from build123d import *

# Parameters (mm, degrees)
EXTRUDE_1_DEPTH     = 30
EXTRUDE_2_DEPTH     = 4
SKETCH_3_R          = 3.25
CUT_EXTRUDE_1_DEPTH = 7
SKETCH_4_W          = 2.5
SKETCH_4_H          = 6
EXTRUDE_3_DEPTH     = 2.5


with BuildPart() as part:
    # Эскиз1 → Бобышка-Вытянуть1 (new body, symmetric)
    with BuildSketch(Plane.XY):
        Polygon((0, 60), (0, 0), (60, 0), (60, 6), (6, 6), (6, 60), align=None)
    extrude(amount=EXTRUDE_1_DEPTH, both=True)

    # Эскиз2 → Бобышка-Вытянуть2 (add)
    with BuildSketch(Plane.XY.offset(30)):
        with BuildLine():
            Line((60, 6), (6, 6))
            Line((6, 6), (6, 60))
            Line((6, 60), (9, 60))
            ThreePointArc((9, 60), (11.121320344, 59.121320344), (12, 57))
            Line((12, 57), (12, 55))
            Line((12, 55), (55, 12))
            Line((55, 12), (57, 12))
            ThreePointArc((57, 12), (59.121320344, 11.121320344), (60, 9))
            Line((60, 9), (60, 6))
        make_face()
    extrude_2 = extrude(amount=-EXTRUDE_2_DEPTH)

    # Зеркальное отражение2: Бобышка-Вытянуть2 across plane
    add(extrude_2.mirror(Plane.XY))

    # Эскиз3 → Вырез-Вытянуть1 (cut, through all)
    with BuildSketch(Plane(origin=(0, 6, 0), x_dir=(1, 0, 0), z_dir=(0, 1, 0))):
        with Locations(Location((45, -15, 0), (0, 0, 270))):  # turned: the seam where the file's is
            Circle(SKETCH_3_R)
        with Locations(Location((45, 15, 0), (0, 0, 90))):  # turned: the seam where the file's is
            Circle(SKETCH_3_R)
        with BuildLine():
            Line((17, -11.75), (31, -11.75))
            ThreePointArc((31, -11.75), (34.25, -15), (31, -18.25))
            Line((31, -18.25), (17, -18.25))
            ThreePointArc((17, -18.25), (13.75, -15), (17, -11.75))
        make_face()
        with BuildLine():
            Line((17, 11.75), (31, 11.75))
            ThreePointArc((31, 11.75), (34.25, 15), (31, 18.25))
            Line((31, 18.25), (17, 18.25))
            ThreePointArc((17, 18.25), (13.75, 15), (17, 11.75))
        make_face()
    cut_extrude_1 = extrude(amount=-CUT_EXTRUDE_1_DEPTH, mode=Mode.SUBTRACT)

    # Эскиз4 → Бобышка-Вытянуть3 (add)
    with BuildSketch(Plane.XZ):
        with Locations((4.25, -15)):
            Rectangle(SKETCH_4_W, SKETCH_4_H)
        with Locations((55.75, -15)):
            Rectangle(SKETCH_4_W, SKETCH_4_H)
        with Locations((55.75, 15)):
            Rectangle(SKETCH_4_W, SKETCH_4_H)
        with Locations((4.25, 15)):
            Rectangle(SKETCH_4_W, SKETCH_4_H)
    extrude_3 = extrude(amount=EXTRUDE_3_DEPTH)

    # Зеркальное отражение3: Вырез-Вытянуть1, Бобышка-Вытянуть3 across plane
    add(cut_extrude_1.mirror(Plane(origin=(0, 0, 0), x_dir=(0, 0, 1), z_dir=(-0.707106781, 0.707106781, 0))), mode=Mode.SUBTRACT)
    add(extrude_3.mirror(Plane(origin=(0, 0, 0), x_dir=(0, 0, 1), z_dir=(-0.707106781, 0.707106781, 0))))


solid = part.part
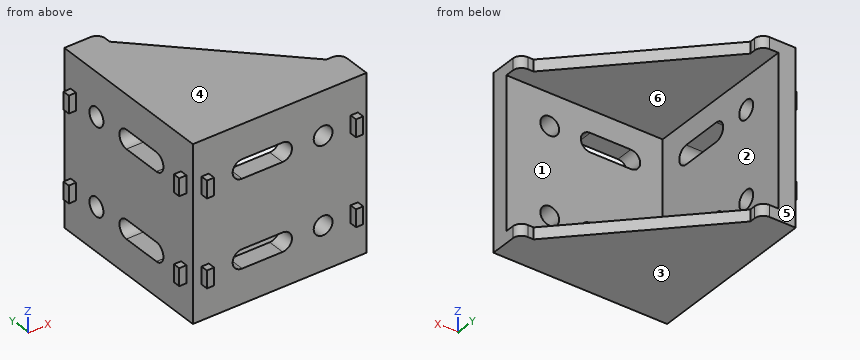
Input: part model. Units: mm. Frame: model coordinates. Face numbers are marked on the shaded views. A direction names the side the tool comes from. Coordinates: 2 decimals unless noted, no trailing zeros. Loops run counter-clockwise (first coordinate to the right, second up) from the corner with the lowest first, then second, coordinate; pieces in that order, holes last. Notation, with made-up numbers: (72.5, 2) - (89.5, 2) arc R18 ccw to (89.5, 26) - close; hole circle Ø4 at (-28.75, 88.25). An arc over 180 degrees is marked (long way). Answer in a Markdown table with one row per item. Add a question column.
Item 1: Section query A-A on x = 45. Return the cut outline in (y, z).
Item 2: Mould query, pull axis Z, two halves, no side actions, for the marked faces 1, 2, 3 and 4. Classes: released by +Z, released by -Z, zero draft, split by the parting line, or undercut.
Item 3: Section query B-B on y = 30. Return the cut outline in (x, z), then the cut area to 3 significant figures.
Item 4: Line query: line 1 along X through (y, z) = (4, 15); line 2 along Y through (x, z) = (2, -15). Output: solid intervals per line, ascending. Write a range as [from, to].
Item 5: Section query D-D on z = 15. State how many separate pieces and enclosed holes the cut face has, then the cut area to 3 significant figures.
Item 6: Section query C-C on y = 2. Return the cut outline in (x, z).
Item 7: Access query for the marked faces 5 and 6. Directions: +Z, -Z, +X, -X, +Y, -Y. A direction counts if a zero-diameter tool reaches every point of the face in a straight line with its end or side. Return the directions, or none.
Item 8: Contact query for flat-ended pins moving along their axis: P1, Ø0.8, axis at x = -1, y = 4, coming from the -Z side; P2, Ø0.8, axis at y = -1.5, z = -14.5, coming from the -X side; P3, Ø6, axis at x = 32.5, z = -10.5, coming from the +Y side. Output: stop coordinate, or through.
Recorded:
| question | item | result |
|---|---|---|
| 1 | outline | (0, -30) - (22, -30) - (22, -26) - (6, -26) - (6, -18.25) - (0, -18.25) - close; (0, -11.75) - (6, -11.75) - (6, 11.75) - (0, 11.75) - close; (0, 18.25) - (6, 18.25) - (6, 26) - (22, 26) - (22, 30) - (0, 30) - close |
| 2 | face 1 | undercut |
| 2 | face 2 | undercut |
| 2 | face 3 | released by -Z |
| 2 | face 4 | released by +Z |
| 3 | outline | (0, -30) - (37, -30) - (37, -26) - (6, -26) - (6, -18.25) - (0, -18.25) - close; (0, -11.75) - (6, -11.75) - (6, 11.75) - (0, 11.75) - close; (0, 18.25) - (6, 18.25) - (6, 26) - (37, 26) - (37, 30) - (0, 30) - close |
| 3 | area | 530 mm^2 |
| 4 | line 1 | [-2.5, 13.75], [34.25, 41.75], [48.25, 60] |
| 4 | line 2 | [0, 13.75], [34.25, 41.75], [48.25, 60] |
| 5 | separate pieces | 5 |
| 5 | enclosed holes | 0 |
| 5 | area | 385 mm^2 |
| 6 | outline | (0, -30) - (60, -30) - (60, 30) - (0, 30) - close; hole (17, -18.25) - (31, -18.25) arc R3.25 ccw to (31, -11.75) - (17, -11.75) arc R3.25 ccw to start; hole (17, 11.75) - (31, 11.75) arc R3.25 ccw to (31, 18.25) - (17, 18.25) arc R3.25 ccw to start; hole circle Ø6.5 at (45, -15); hole circle Ø6.5 at (45, 15) |
| 7 | face 5 | +Z, -Z, +X, -X, +Y |
| 7 | face 6 | +X, +Y |
| 8 | P1 | z = -18 |
| 8 | P2 | x = 3 |
| 8 | P3 | y = 6 |
